Answer from the drawing. Dimensions are ordinates in mm from the lowest x, y and z of the part. A direction names the side the tool comes from. Coordinates: 2 decimals unless noted, no trailing zeros. Write each loop counter-clockwise with the first axis right and the second up, starting at its lowest first coordinate (ties: lowest second). Pieces come first, ordered by that corner, then holes. Notation, with made-up numbers: (-17, -39) -> (15, -39) arc R22 ccw to (15, -13) -> close; hole circle Ø7 at (-24.5, -4.5). An arc over 180 degrees is marked (long way). One line per item, written item: value. Start each with the question number.
1. Given P1, Ø6, axis at y = 7, z = 25.5, coming from the -X side; P2, Ø1.5, axis at x = 1.5, y = 5, coming from the +Z side; P3, Ø2, axis at x = 19, y = 4, coming from the +Z side, each flat-ended and moving along its own axis, determine where each tip first touches the part or whether it passes through.
2. Find section A-A, the plane x = 10.8. Write down the section's boundary in (y, z).
3. Consider line 1 along Z through (x, y) = (11, 0.5); line 2 along X through (y, z) = (3, 13); line 3 along Z through (x, y) = (1, 2.75). Determine where each line is inside the solid, lowest interval first.
4. Find section B-B, the plane y = 0.5. Write down the section's boundary in (x, z).
5. Find section D-D, the plane y = 6.1. Write down the section's boundary in (x, z).
6. Find section C-C, the plane z = 18. Write down the section's boundary in (x, y), and give its area (3 significant figures).
7. For the marked faces 1, 2, 3 and 4, determine the directions among +Z, -Z, +X, -X, +Y, -Y from which every point of the face is accessible in a straight line to the end or side of a thin tool.
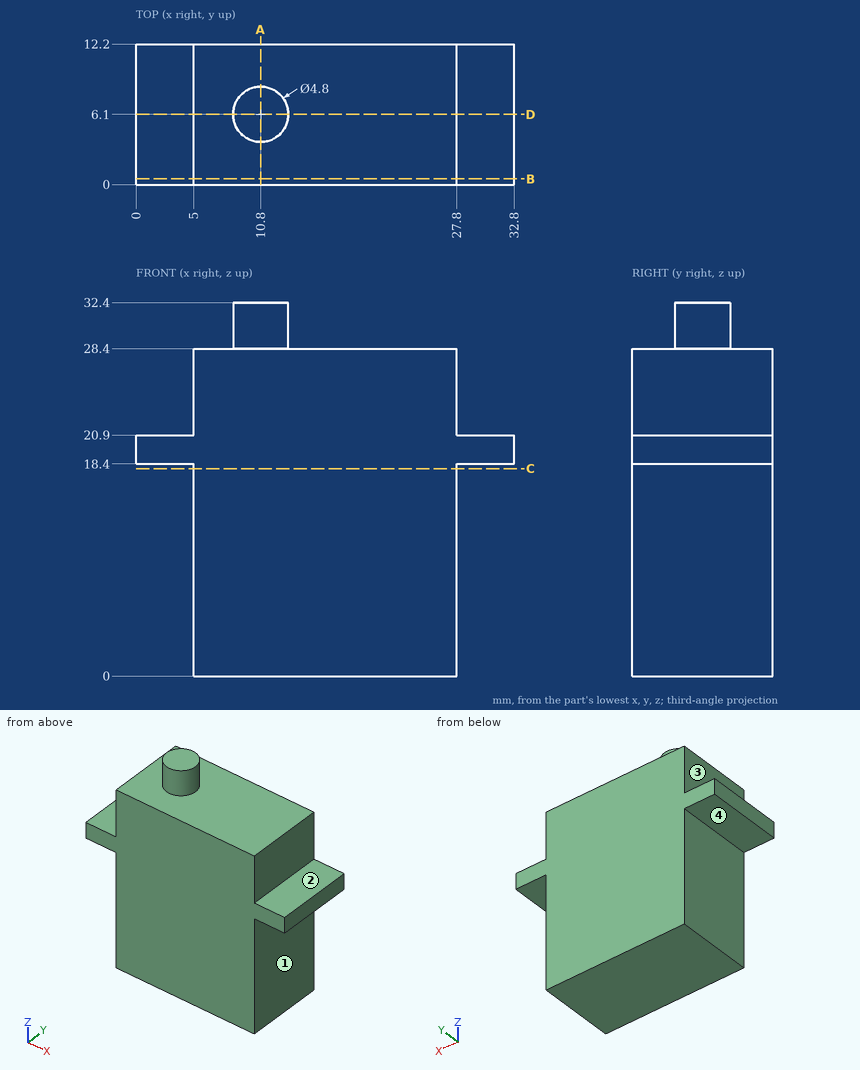
Answer block:
1. P1: stops at x = 5
1. P2: stops at z = 20.9
1. P3: stops at z = 28.4
2. outline: (0, 0) -> (12.2, 0) -> (12.2, 28.4) -> (8.5, 28.4) -> (8.5, 32.4) -> (3.7, 32.4) -> (3.7, 28.4) -> (0, 28.4) -> close
3. line 1: z = 0 to 28.4
3. line 2: x = 5 to 27.8
3. line 3: z = 18.4 to 20.9
4. outline: (0, 18.4) -> (5, 18.4) -> (5, 0) -> (27.8, 0) -> (27.8, 18.4) -> (32.8, 18.4) -> (32.8, 20.9) -> (27.8, 20.9) -> (27.8, 28.4) -> (5, 28.4) -> (5, 20.9) -> (0, 20.9) -> close
5. outline: (0, 18.4) -> (5, 18.4) -> (5, 0) -> (27.8, 0) -> (27.8, 18.4) -> (32.8, 18.4) -> (32.8, 20.9) -> (27.8, 20.9) -> (27.8, 28.4) -> (13.2, 28.4) -> (13.2, 32.4) -> (8.4, 32.4) -> (8.4, 28.4) -> (5, 28.4) -> (5, 20.9) -> (0, 20.9) -> close
6. outline: (5, 0) -> (27.8, 0) -> (27.8, 12.2) -> (5, 12.2) -> close
6. area: 278 mm2
7. face 1: -Z, +X, +Y, -Y
7. face 2: +Z, +X, +Y, -Y
7. face 3: +Z, -X, +Y, -Y
7. face 4: -Z, -X, +Y, -Y
